Can you work these out from the model? Positions are in its coordinate system, mm. Round coordinates to 2 decimals unless told otherwise and drop trailing zeros. Write each loop counter-clockwise with the first axis right and the second up, starting at its lowest first coordinate (ties: lowest second). Pieces come first, ordered by that corner, then holes.
Q1. Please list where these lines run through material, in increasing order: line 1 along Z through (x, y) = (-2, 28); line 2 along Z through (x, y) = (3.75, 17); line 3 along Y through (x, z) = (-3.5, -0.5).
Q2. If we section it at B-B (z = 13.5): Please give me the cut outline in (x, y).
Q3. If we section it at A-A (y = 0): Please give me the cut outline in (x, z).
Q4. I'm going to push flat-ended pins straight in: pin 1 Ø8 at (y, z) = (10, 6) entering from -X; pin 2 Ø5 at (x, y) = (-3, 19.5) entering from +Z; pin 3 Ø2 at (x, z) = (1, 6) entering from -Y. Where does each tip first touch, or does it pass through?
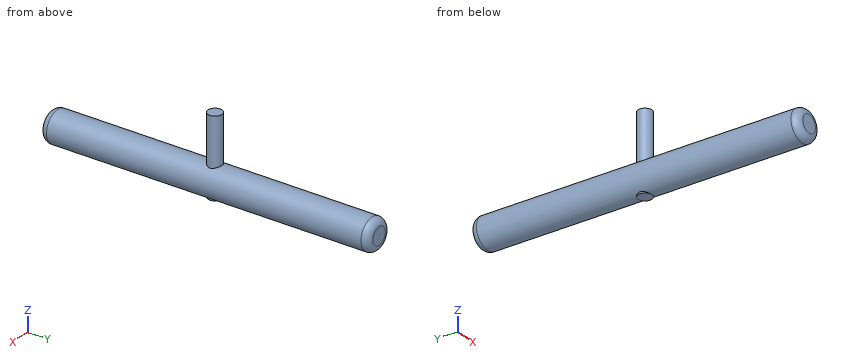
Autodesk Inventor part; units mm, degrees
ref_plane "YZ Plane" through (0, 0, 0) normal (1, 0, 0) x (0, 1, 0)
ref_plane "XZ Plane" through (0, 0, 0) normal (0, 1, 0) x (-1, 0, 0)
ref_plane "XY Plane" through (0, 0, 0) normal (0, 0, 1) x (1, 0, 0)
sketch "Sketch1" plane through (0, 0, 0) normal (0, 1, 0) x (-1, 0, 0)
  circle A0 centre (0, 0) radius 4.5
  dimension "d0" = 9
extrude "Extrusion1" add sketch "Sketch1" along normal mid plane 95
fillet "Fillet1" radius 2 2 edges at (4.5, 47.5, 0) (4.5, -47.5, 0)
sketch "Sketch2" plane through (0, 0, 0) normal (0, 0, 1) x (1, 0, 0)
  circle A0 centre (0, 0) radius 2
  dimension "d4" = 4
extrude "Extrusion2" add sketch "Sketch2" along normal blind 18 and the other way blind 4.5
properties part number "Part2pasador" material "Steel"
A:
1. line 1: z = -4.03 to 4.03
1. line 2: z = -2.49 to 2.49
1. line 3: y = -47.21 to 47.21
2. outline: circle Ø4 at (0, 0)
3. outline: (-2, -4.5) - (2, -4.5) - (2, -4.03) arc R4.5 ccw to (2, 4.03) - (2, 18) - (-2, 18) - (-2, 4.03) arc R4.5 ccw to (-2, -4.03) - close
4. pin 1: stops at x = -4.03
4. pin 2: stops at z = 4.47
4. pin 3: stops at y = -2
